```python
from build123d import *

# Parameters (mm, degrees)
CROQUIS1_R              = 11
CROQUIS1_R_2            = 6.5
SALIENTE_EXTRUIR2_DEPTH = 1
CROQUIS1_6_R            = 9.1
CROQUIS1_6_R_2          = 8.1
SALIENTE_EXTRUIR3_DEPTH = 2.5
CROQUIS1_8_R            = 12
CROQUIS1_8_R_2          = 11
SALIENTE_EXTRUIR4_DEPTH = 10
CROQUIS10_W             = 5
CROQUIS10_H             = 5
CORTAR_EXTRUIR1_DEPTH   = 30


with BuildPart() as part:
    # Croquis1 → Saliente-Extruir2 (new body)
    with BuildSketch(Plane(origin=(0, 0, 0), x_dir=(1, 0, 0), z_dir=(0, 1, 0))):
        with Locations((8.8, 6.6)):
            Circle(CROQUIS1_R)
        with Locations((8.8, 6.6)):
            Circle(CROQUIS1_R_2, mode=Mode.SUBTRACT)
    extrude(amount=SALIENTE_EXTRUIR2_DEPTH)

    # Croquis1_6 → Saliente-Extruir3 (add)
    with BuildSketch(Plane(origin=(0, 0, 0), x_dir=(1, 0, 0), z_dir=(0, 1, 0))):
        with Locations((8.8, 6.6)):
            Circle(CROQUIS1_6_R)
        with Locations((8.8, 6.6)):
            Circle(CROQUIS1_6_R_2, mode=Mode.SUBTRACT)
    extrude(amount=SALIENTE_EXTRUIR3_DEPTH)

    # Croquis1_8 → Saliente-Extruir4 (add)
    with BuildSketch(Plane(origin=(0, 0, 0), x_dir=(1, 0, 0), z_dir=(0, 1, 0))):
        with Locations((8.8, 6.6)):
            Circle(CROQUIS1_8_R)
        with Locations((8.8, 6.6)):
            Circle(CROQUIS1_8_R_2, mode=Mode.SUBTRACT)
    extrude(amount=SALIENTE_EXTRUIR4_DEPTH)

    # Croquis10 → Cortar-Extruir1 (cut)
    with BuildSketch(Plane.XY):
        with Locations((11.3, 5)):
            Rectangle(CROQUIS10_W, CROQUIS10_H)
        with Locations((6.3, 5)):
            Rectangle(CROQUIS10_W, CROQUIS10_H)
    extrude(amount=CORTAR_EXTRUIR1_DEPTH, mode=Mode.SUBTRACT)


solid = part.part
```
Can you work these out from the model? Positions are in its coordinate system, mm. A direction names the side the tool comes from. Coordinates: 2 decimals unless noted, no trailing zeros. Loops run counter-clockwise (first coordinate to the right, second up) from the corner with the lowest first, then second, coordinate; pieces in that order, holes last.
1) Imagine slicing it at D-D on y = 7. List the corners of the cut face in (x, z) for me, plus the area to 3 significant figures.
2) Imagine slicing it at C-C on y = 8.75. List the corners of the cut face in (x, z) for me.
3) Which directions (+Z, -Z, +X, -X, +Y, -Y) give clear straight access to the entire face, cutting with the end or side of a thin tool? Please do faces 1 (the flat face through (13.8, 5, 4)), 2 (the flat face through (19, 10, -1)), 3 (the cylindrical face through (14.714, 5.437, -15.875)).
4) Imagine slicing it at B-B on z = -6.6. List the corners of the cut face in (x, y) for me.
5) Thinking about a two-plate mould opening in Y: for faces 4 (the flat face through (14, 0, -1)), 5 (the cylindrical face through (1.58, 1.74, -1.06)), 6 (the flat face through (3.8, 5, 4)), which applies, pulls with the +Y half, pulls with the -Y half, needs draft (parallel to the pull), parting line crosses it, or undercut?
6) For pin 1 (5 mm diameter, centred on x = 5.5, z = -5.5, fed in from +Y); pin 2 (1 mm diameter, centred on x = 15.5, z = 1, fed in from +Y); pin 3 (1.2 mm diameter, centred on y = 6, z = 3.5, fed in from +X); pin 4 (10 mm diameter, centred on x = 5.5, z = -5, fed in from +Y), each with a flat end and sliding along its axis, tell me the tip position at first contact or that it passes through.
7) I need wall thicknesses on probe 1 along X at (y, z) = (5.5, -6.6); probe 2 along Z at (x, y) = (8.8, 0.4); probe 3 along X at (y, z) = (1.75, 1.75). Which ranges of each line are inside material? Lowest first, please.
8) Imagine slicing it at A-A on x = 8.8. List the corners of the cut face in (y, z) for me.
Completed:
1. outline: (3.8, 3.2) - (3.8, 4.31) arc R12 ccw (long way) to (13.8, 4.31) - (13.8, 3.2) arc R11 cw (long way) to start
1. area: 61.9 mm2
2. outline: circle Ø24 at (8.8, -6.6); hole circle Ø22 at (8.8, -6.6)
3. face 1: +Z
3. face 2: +Z, -Z, +X, -X, +Y
3. face 3: +Y
4. outline: (-3.2, 0) - (2.3, 0) - (2.3, 1) - (0.7, 1) - (0.7, 2.5) - (-0.3, 2.5) - (-0.3, 1) - (-2.2, 1) - (-2.2, 10) - (-3.2, 10) - close; (15.3, 0) - (20.8, 0) - (20.8, 10) - (19.8, 10) - (19.8, 1) - (17.9, 1) - (17.9, 2.5) - (16.9, 2.5) - (16.9, 1) - (15.3, 1) - close
5. face 4: pulls with the -Y half
5. face 5: needs draft
5. face 6: undercut
6. pin 1: passes through
6. pin 2: stops at y = 1
6. pin 3: stops at x = 16.13
6. pin 4: stops at y = 2.5
7. probe 1: x = -3.2 to -2.2, 19.8 to 20.8
7. probe 2: z = -18.6 to -13.1, -0.1 to 5.4
7. probe 3: x = 0.18 to 1.64, 5.18 to 12.42, 15.96 to 17.42
8. outline: (0, -18.6) - (10, -18.6) - (10, -17.6) - (1, -17.6) - (1, -15.7) - (2.5, -15.7) - (2.5, -14.7) - (1, -14.7) - (1, -13.1) - (0, -13.1) - close; (0, -0.1) - (1, -0.1) - (1, 1.5) - (2.5, 1.5) - (2.5, 2.5) - (1, 2.5) - (1, 4.4) - (2.5, 4.4) - (2.5, 5.4) - (0, 5.4) - close; (7.5, 4.4) - (10, 4.4) - (10, 5.4) - (7.5, 5.4) - close
